Answer from the drawing. Dimensions are ordinates in mm from the lowest x, y and z of the part. A direction names the side the tool comes from. Coordinates: 2 decimals unless noted, no trailing zeros. Write each loop counter-clockwise with the first axis right and the second up, starting at its lowest first coordinate (ties: lowest second). Pieces come first, ordered by that corner, then holes.
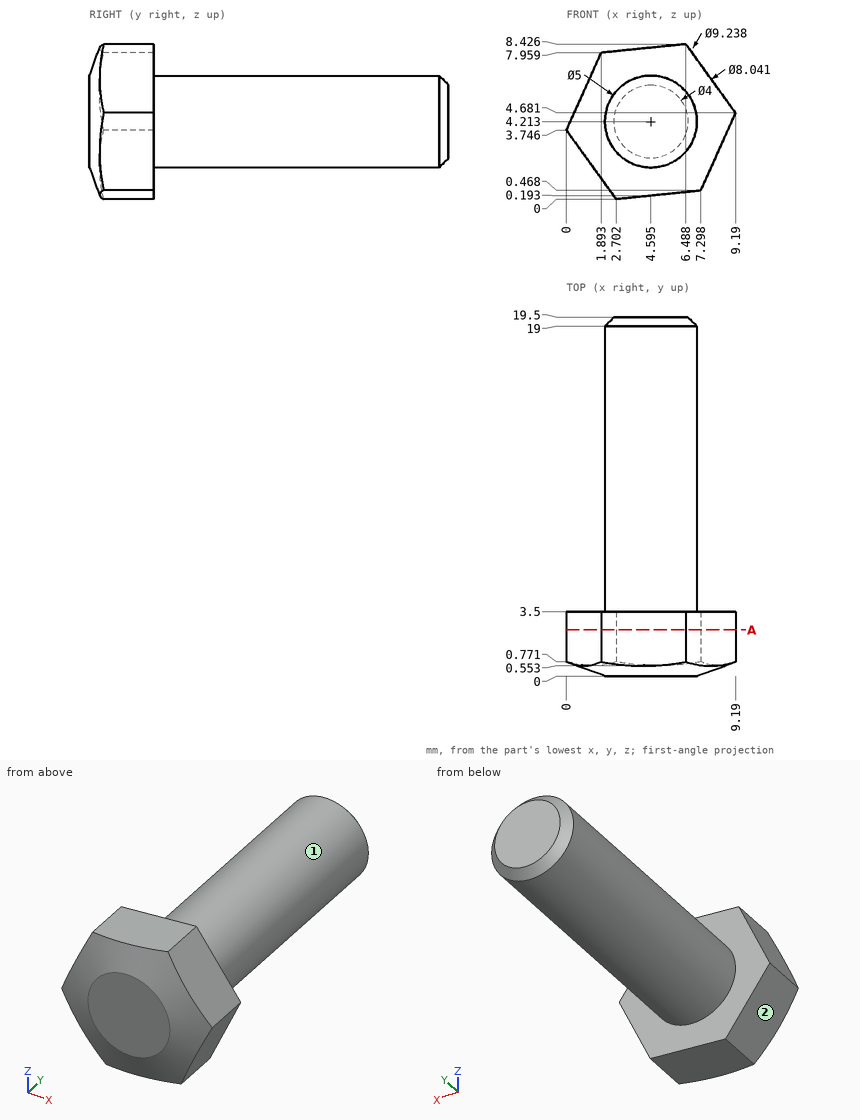
(1) Each of these flat-tipped pins is pushed along its axis until it touches: pin 1 (4 mm diameter, centred on y = 14.5, z = 1, fed in from +X); pin 2 (2 mm diameter, centred on x = 1.5, y = 7, fed in from -Z); pin 3 (1 mm diameter, centred on x = 1, z = 3, fed in from +Y). Where does it stop, or does it pass through?
(2) Section A-A, the plane y = 2.5 is taken. Write down the section's boundary in (x, z) (1 decimal).
(3) Which of the six approach directions +Z, -Z, +X, -X, +Y, -Y give full straight-line access (tool end or side, diameter ignored) to the marked faces 1 and 2?
(4) Find the intervals of material crossed by probe 1 along X at (y, z) = (8, 4.25) (1 decimal); probe 2 along X at (y, z) = (8, 6.25) (1 decimal); probe 3 along Z at (x, y) = (4, 14.5) (1 decimal), in increasing order.
Solution:
1. pin 1: stops at x = 6.78
1. pin 2: stops at z = 2.85
1. pin 3: stops at y = 3.5
2. outline: (0, 3.7) - (2.7, 0) - (7.3, 0.5) - (9.2, 4.7) - (6.5, 8.4) - (1.9, 8) - close
3. face 1: +Y
3. face 2: -Z, -X, +Y, -Y
4. probe 1: x = 2.1 to 7.1
4. probe 2: x = 3.1 to 6
4. probe 3: z = 1.8 to 6.6
